Autodesk Inventor part; units mm, degrees
ref_plane "YZ Plane" through (0, 0, 0) normal (1, 0, 0) x (0, 1, 0)
ref_plane "XZ Plane" through (0, 0, 0) normal (0, 1, 0) x (-1, 0, 0)
ref_plane "XY Plane" through (0, 0, 0) normal (0, 0, 1) x (1, 0, 0)
sketch "Sketch1" plane through (0, 0, 0) normal (0, 1, 0) x (-1, 0, 0)
  line L0 (-21, 21) -> (21, 21)
  line L1 (21, 21) -> (21, -21)
  line L2 (21, -21) -> (-21, -21)
  line L3 (-21, -21) -> (-21, 21)
  line L4 (-21, 21) -> (21, -21) construction
  line L5 (21, 21) -> (-21, -21) construction
  point P0 (0, 0)
  dimension "d0" = 42
  dimension "d1" = 42
extrude "Extrusion1" add sketch "Sketch1" along normal blind 60
sketch "Sketch2" plane through (0, 60, 0) normal (0, 1, 0) x (1, 0, 0)
  circle A0 centre (0, 0) radius 17.25
  dimension "d4" = 34.5
extrude "Extrusion2" cut sketch "Sketch2" against normal through all
sketch "Sketch3" plane through (0, 60, 0) normal (0, 1, 0) x (1, 0, 0)
  circle A0 centre (0, 0) radius 19.25
  dimension "d7" = 38.5
extrude "Extrusion3" cut sketch "Sketch3" against normal blind 20
sketch "Sketch4" plane through (21, 0, -21) normal (0, 0, -1) x (-1, 0, 0)
  line L0 (16, -5) -> (26, -5)
  line L1 (26, -5) -> (26, 5)
  line L2 (26, 5) -> (16, 5)
  line L3 (16, 5) -> (16, -5)
  line L4 (16, -5) -> (26, 5) construction
  line L5 (26, -5) -> (16, 5) construction
  point P0 (21, 0)
  dimension "d10" = 10
  dimension "d11" = 10
extrude "Extrusion4" cut sketch "Sketch4" against normal through all
properties part number "DCMotorHolder"
Source: CAD feature listing. Evaluate the final solid. Frame: model axes, mm. A direction names the side the tool comes from. Round coordinates to 2 decimals unless told otherwise and drop trailing zeros. Write each loop counter-clockwise with the first axis right and the second up, starting at its lowest first coordinate (ties: lowest second). Pieces come first, ordered by that corner, then holes. Notation, with made-up numbers: (-38, -26) - (-19, -26) arc R23 cw to (-19, -10) - close; hole circle Ø5 at (-33, 32.5). An arc over 180 degrees is marked (long way). Use CSV: the item, a comma, the result in double quotes. Start each with the question number.
(1) Material intervals for probe 1 along Z at (x, y) = (0, 54.5); probe 2 along X at (y, z) = (5.5, 5), sorted ascending. Write a range as [from, to].
(2) Set-up query: faces 4 (the face through (5, 3, 19)), 5 (the face through (-16, 40, -7)), 6 (the face through (18, 0, 0)). Return all of +Z, -Z, +X, -X, +Y, -Y with unobstructed straight access to the full face (end or side cutting, diameter ignored); none if empty.
(3) Cut plane C-C, the plane y = 42.5. Return loops of the section in (x, z).
(4) First-contact query: pin 1 Ø12 at (x, z) = (4, -5.5) entering from -Y; pin 2 Ø4 at (x, z) = (-10.5, -11.5) entering from +Y; pin 3 Ø1.3 at (x, z) = (0, -18.5) entering from -Y. Flat tips, straight axial feed; report the tip coordinate or a pass-through.
(5) Cut plane B-B, the plane x = 0. Return loops of the section in (y, z).
(6) Cut plane D-D, the plane y = 6.5. Return loops of the section in (x, z), and give its area (3 significant figures).
(7) Cut plane A-A, the plane z = 0. Return loops of the section in (x, y).
(8) Mould query, pull axis Z, two halves, no side actions, for faces 1 (the face through (5, 3, -19)), 2 (the face through (-15.28, 50.14, 11.71)), 3 (the face through (0, 30, -21)). Classes: pulls with the +Z half, pulls with the -Z half, needs draft (parallel to the pull), parting line crosses it, or undercut.
Geometry says:
1,probe 1,"[-21, -19.25], [19.25, 21]"
1,probe 2,"[-21, -16.51], [16.51, 21]"
2,face 4,"+Z, -Z, -Y"
2,face 5,"+Y"
2,face 6,"+Z, -Z, +X, -X, -Y"
3,outline,"(-21, -21) - (21, -21) - (21, 21) - (-21, 21) - close; hole circle Ø38.5 at (0, 0)"
4,pin 1,"through"
4,pin 2,"y = 40"
4,pin 3,"y = 5"
5,outline,"(5, -21) - (60, -21) - (60, -19.25) - (40, -19.25) - (40, -17.25) - (5, -17.25) - close; (5, 17.25) - (40, 17.25) - (40, 19.25) - (60, 19.25) - (60, 21) - (5, 21) - close"
6,outline,"(-21, -21) - (21, -21) - (21, 21) - (-21, 21) - close; hole circle Ø34.5 at (0, 0)"
6,area,"829 mm²"
7,outline,"(-21, 0) - (-17.25, 0) - (-17.25, 40) - (-19.25, 40) - (-19.25, 60) - (-21, 60) - close; (17.25, 0) - (21, 0) - (21, 60) - (19.25, 60) - (19.25, 40) - (17.25, 40) - close"
8,face 1,"needs draft"
8,face 2,"undercut"
8,face 3,"pulls with the -Z half"
